Check sheet for the modelled part. Datum: model origin and axes. Units: mm. Coordinates: 2 decimals unless noted, no trailing zeros. Loops run counter-clockwise (first coordinate to the right, second up) from the corner with the lowest first, then second, coordinate; pieces in that order, holes last.
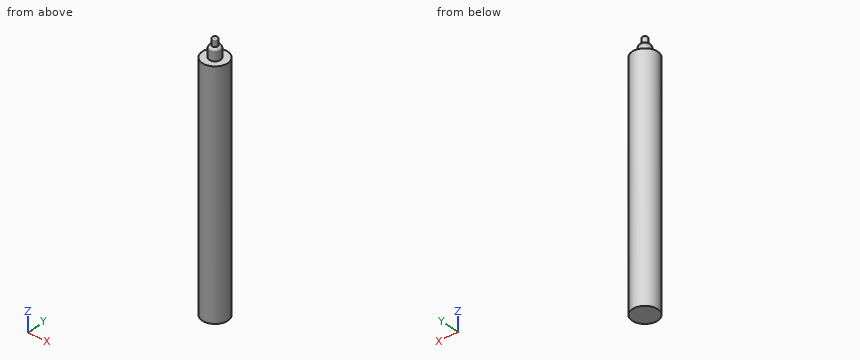
```python
from build123d import *

# Parameters (mm, degrees)
SKETCH_1_R      = 9
EXTRUDE_1_DEPTH = 167
SKETCH_2_R      = 4
EXTRUDE_2_DEPTH = 8
SKETCH_3_R      = 2
EXTRUDE_3_DEPTH = 5
FILLET_1_R      = 2
FILLET_2_R      = 1


with BuildPart() as part:
    # Эскиз1 → Бобышка-Вытянуть1 (new body)
    with BuildSketch(Plane.XY):
        with Locations(Location((0, 0, 0), (0, 0, 180))):
            Circle(SKETCH_1_R)
    extrude(amount=EXTRUDE_1_DEPTH)

    # Эскиз2 → Бобышка-Вытянуть2 (add)
    with BuildSketch(Plane.XY.offset(167)):
        Circle(SKETCH_2_R)
    extrude(amount=EXTRUDE_2_DEPTH)

    # Эскиз3 → Бобышка-Вытянуть3 (add)
    with BuildSketch(Plane.XY.offset(175)):
        Circle(SKETCH_3_R)
    extrude(amount=EXTRUDE_3_DEPTH)

    # Скругление1
    fillet_1_edges = [part.edges().sort_by_distance(p)[0] for p in [
        (-4, 0, 175),
    ]]
    fillet(fillet_1_edges, radius=FILLET_1_R - 0.0001)  # a hair under: the kernel refuses the full size

    # Скругление2
    fillet_2_edges = [part.edges().sort_by_distance(p)[0] for p in [
        (-2, 0, 180),
    ]]
    fillet(fillet_2_edges, radius=FILLET_2_R)


solid = part.part
```
1) Section check A-A on z = 114.5. Enter the section's corners in (x, y), plus the area to 3 significant figures.
Answer sheet:
outline: circle Ø18 at (0, 0)
area: 254 mm2
2) Depth check by flat-ended pin: pin 1 (10 mm diameter, centred on y = -5.5, z = 109, fed in from -X); pin 2 (1.5 mm diameter, centred on y = 5, z = 133, fed in from +X); pin 3 (6 mm diameter, centred on y = 5.5, z = 43.5, fed in from +X). Enter the tip coordinate at first touch or a pass-through.
Answer sheet:
pin 1: stops at x = -8.99
pin 2: stops at x = 7.93
pin 3: stops at x = 8.65
3) Scan lines: line 1 (X direction, y = 0.75, z = 15); line 2 (Z direction, x = -5.25, y = -3.5); line 3 (Y direction, x = 0.5, z = 135). Record each from-to range of solid material in increasing order.
Answer sheet:
line 1: x = -8.97 to 8.97
line 2: z = 0 to 167
line 3: y = -8.99 to 8.99
4) Section check C-C on x = -6.25. Enter the section's corners in (y, z), plus the area to 3 significant figures.
Answer sheet:
outline: (-6.48, 0) - (6.48, 0) - (6.48, 167) - (-6.48, 167) - close
area: 2,160 mm2
5) Section check B-B on y = -6. Enter the section's corners in (x, z).
Answer sheet:
outline: (-6.71, 0) - (6.71, 0) - (6.71, 167) - (-6.71, 167) - close
